Here's how the part is built. I have some questions about the finished solid (model axes, mm). A direction names the side the tool comes from. Round coordinates to 2 decimals unless told otherwise and drop trailing zeros. Write each loop counter-clockwise with the first axis right and the second up, starting at its lowest first coordinate (ties: lowest second). Pieces come first, ordered by that corner, then holes. Notation, with made-up numbers: M 68.25,59.25 L 99.25,59.25 A34 ccw 99.25,89.25 Z; hole C 16.5,75.5 d7. An arc over 180 degrees is marked long. Use a Markdown table: item, result. Add a question column.
```python
from build123d import *

# Parameters (mm, degrees)
SKETCH_R     = 8.4
PAD_DEPTH    = 8
SKETCH001_R  = 1.5
PAD001_DEPTH = 3
POCKET_DEPTH = 25.001


with BuildPart() as part:
    # Sketch → Pad (new body)
    with BuildSketch(Plane.XZ):
        with BuildLine():
            Line((-13, 22), (13, 22))
            ThreePointArc((22.5, 12.5), (19.717514, 19.217514), (13, 22))
            Line((22.5, 12.5), (22.5, 0))
            Line((22.5, 0), (-22.5, 0))
            Line((-22.5, 0), (-22.5, 12.5))
            ThreePointArc((-13, 22), (-19.717514, 19.217514), (-22.5, 12.5))
        make_face()
        with Locations((-13, 12.5)):
            Circle(SKETCH_R, mode=Mode.SUBTRACT)
        with Locations((13, 12.5)):
            Circle(SKETCH_R, mode=Mode.SUBTRACT)
        with BuildLine():
            ThreePointArc((-2.822, 7.336), (-5, 5.158), (-2.822, 2.98))
            Line((-2.822, 2.98), (2.822, 2.98))
            ThreePointArc((2.822, 2.98), (5, 5.158), (2.822, 7.336))
            Line((2.822, 7.336), (-2.822, 7.336))
        make_face(mode=Mode.SUBTRACT)
    extrude(amount=PAD_DEPTH)

    # Sketch001 (on Face2 of Pad) → Pad001 (join)
    with BuildSketch(Plane(origin=(0, 0, 0), x_dir=(1, 0, 0), z_dir=(0, 0, -1))):
        with BuildLine():
            Line((-9, -12), (9, -12))
            ThreePointArc((9, -12), (11.12132, -11.12132), (12, -9))
            Line((12, -9), (12, 8))
            Line((12, 8), (-12, 8))
            Line((-12, 8), (-12, -9))
            ThreePointArc((-12, -9), (-11.12132, -11.12132), (-9, -12))
        make_face()
        with Locations((-8, -6.5)):
            Circle(SKETCH001_R, mode=Mode.SUBTRACT)
        with Locations((8, -6.5)):
            Circle(SKETCH001_R, mode=Mode.SUBTRACT)
    extrude(amount=PAD001_DEPTH)

    # Sketch002 (on Face6 of Pad001) → Pocket (cut, through all)
    with BuildSketch(Plane.XY.offset(22)):
        with BuildLine():
            Line((-22.5, -2), (-22.5, -9))
            Line((-22.5, -9), (22.5, -9))
            Line((22.5, -9), (22.5, -2))
            ThreePointArc((-22.5, -2), (0, -8), (22.5, -2))
        make_face()
    extrude(amount=-POCKET_DEPTH, mode=Mode.SUBTRACT)


solid = part.part
```
Item 1: Imagine slicing it at C-C on x = -18. List the corners of the cut face in (y, z) for me, plus the area to 3 significant figures.
Item 2: Imagine slicing it at B-B on z = 15.75. List the corners of the cut face in (x, y) for me (1 decimal), plus the area to 3 significant figures.
Item 3: On a 3-axis mill with a long thin cutter (end or side, diameter ignored), from which of +Z, -Z, +X, -X, +Y, -Y can I reach the whole of each face in a straight line? I mean faces 1 (the face through (16, -2, 0)), 2 (the face through (5, -3.9, 5.1)), 3 (the face through (-16, -2, 0)), 4 (the face through (0, 2, -3)). Say none if no direction works.
Item 4: For pin 1 Ø3.5 at (x, y) = (-5.5, 5.5) entering from +Z; pin 2 Ø2.5 at (y, z) = (0, -1.5) entering from -X; pin 3 Ø6 at (y, z) = (-5.5, 2) entering from -X; pin 4 Ø5 at (x, y) = (8, 6.5) entering from -Z, each with a flat end and sliding along its axis, tell me the tip position at first contact or that it passes through.
Item 5: Imagine slicing it at A-A on y = 6.5. List the corners of the cut face in (x, z) for me.
Item 6: I need wall thicknesses on probe 1 along X at (y, z) = (6.5, -1.4); probe 2 along Z at (x, y) = (-13, -2.25); probe 3 along X at (y, z) = (-2.75, 12.25). Which ranges of each line are inside material? Lowest first, please. Write a range as from..to.
Item 7: If we mould it in two halves opening along X, with no side actions, what happens to faces 5 (the face through (0, 0, 11)), 6 (the face through (0, -4, 2.98)), 7 (the face through (-11.14, 11.1, -1.48)), 8 (the face through (0, -8, 10))? For each: +X half, -X half, draft (parallel to the pull), parting line (faces both ways), or undercut.
Item 8: Imagine slicing it at D-D on x = 8. List the corners of the cut face in (y, z) for me, plus the area to 3 significant figures.
The answers:
| question | item | result |
|---|---|---|
| 1 | outline | M -4.26,0 L 0,0 L 0,5.75 L -4.26,5.75 Z; M -4.26,19.25 L 0,19.25 L 0,20.58 L -4.26,20.58 Z |
| 1 | area | 30.2 mm² |
| 2 | outline | M -21.9,-2.3 A45.2 ccw -20.7,-3 L -20.7,0 L -21.9,0 Z; M -5.3,-7.7 A45.2 ccw 5.3,-7.7 L 5.3,0 L -5.3,0 Z; M 20.7,-3 A45.2 ccw 21.9,-2.3 L 21.9,0 L 20.7,0 Z |
| 2 | area | 89.2 mm² |
| 3 | face 1 | -Z, +X, +Y, -Y |
| 3 | face 2 | +Y, -Y |
| 3 | face 3 | -Z, -X, +Y, -Y |
| 3 | face 4 | -Z, +X, -X, +Y, -Y |
| 4 | pin 1 | z = 0 |
| 4 | pin 2 | x = -12 |
| 4 | pin 3 | x = -21.61 |
| 4 | pin 4 | z = -3 |
| 5 | outline | M -12,-3 L -9.5,-3 L -9.5,0 L -12,0 Z; M -6.5,-3 L 6.5,-3 L 6.5,0 L -6.5,0 Z; M 9.5,-3 L 12,-3 L 12,0 L 9.5,0 Z |
| 6 | probe 1 | -12..-9.5, -6.5..6.5, 9.5..12 |
| 6 | probe 2 | 0..4.1, 20.9..22 |
| 6 | probe 3 | -4.6..4.6 |
| 7 | face 5 | draft |
| 7 | face 6 | undercut |
| 7 | face 7 | -X half |
| 7 | face 8 | parting line |
| 8 | outline | M -7.29,-3 L 5,-3 L 5,0 L 0,0 L 0,5.75 L -7.29,5.75 Z; M -7.29,19.25 L 0,19.25 L 0,22 L -7.29,22 Z; M 8,-3 L 12,-3 L 12,0 L 8,0 Z |
| 8 | area | 111 mm² |
